```python
from build123d import *

# Parameters (mm, degrees)
SKETCH1_W                                           = 60
SKETCH1_H                                           = 100
BOSS_EXTRUDE1_DEPTH                                 = 8
CBORE_FOR_M6_HEX_SOCKET_HEAD_CAP_SCREW1_D           = 6.6
CBORE_FOR_M6_HEX_SOCKET_HEAD_CAP_SCREW1_CBORE_D     = 11
CBORE_FOR_M6_HEX_SOCKET_HEAD_CAP_SCREW1_CBORE_DEPTH = 6.4
SKETCH6_R                                           = 14.05
CUT_EXTRUDE1_DEPTH                                  = 61.464865831
SKETCH7_W                                           = 60
SKETCH7_H                                           = 16
BOSS_EXTRUDE2_DEPTH                                 = 32
CBORE_FOR_M6_HEX_SOCKET_HEAD_CAP_SCREW2_D           = 6.6
CBORE_FOR_M6_HEX_SOCKET_HEAD_CAP_SCREW2_CBORE_D     = 11
CBORE_FOR_M6_HEX_SOCKET_HEAD_CAP_SCREW2_CBORE_DEPTH = 6.4


with BuildPart() as part:
    # Sketch1 → Boss-Extrude1 (new, symmetric)
    with BuildSketch(Plane.XY):
        Rectangle(SKETCH1_W, SKETCH1_H)
    extrude(amount=BOSS_EXTRUDE1_DEPTH, both=True)

    # CBORE for M6 Hex Socket Head Cap Screw1 (through all)
    with Locations(Plane.XY.offset(8)):
        with Locations((-20, 40), (20, 40), (20, 0), (-20, 0)):
            CounterBoreHole(CBORE_FOR_M6_HEX_SOCKET_HEAD_CAP_SCREW1_D / 2, CBORE_FOR_M6_HEX_SOCKET_HEAD_CAP_SCREW1_CBORE_D / 2, CBORE_FOR_M6_HEX_SOCKET_HEAD_CAP_SCREW1_CBORE_DEPTH)

    # Sketch6 → Cut-Extrude1 (cut, through all)
    with BuildSketch(Plane.XY.offset(8)):
        with Locations((0, 20)):
            Circle(SKETCH6_R)
    extrude(amount=-CUT_EXTRUDE1_DEPTH, mode=Mode.SUBTRACT)

    # Sketch7 → Boss-Extrude2 (add)
    with BuildSketch(Plane.XY.offset(8)):
        with Locations((0, -42)):
            Rectangle(SKETCH7_W, SKETCH7_H)
    extrude(amount=BOSS_EXTRUDE2_DEPTH)

    # CBORE for M6 Hex Socket Head Cap Screw2 (through all)
    with Locations(Plane(origin=(0, -34, 0), x_dir=(1, 0, 0), z_dir=(0, 1, 0))):
        with Locations((-20, -18), (20, -18), (20, -33), (-20, -33)):
            CounterBoreHole(CBORE_FOR_M6_HEX_SOCKET_HEAD_CAP_SCREW2_D / 2, CBORE_FOR_M6_HEX_SOCKET_HEAD_CAP_SCREW2_CBORE_D / 2, CBORE_FOR_M6_HEX_SOCKET_HEAD_CAP_SCREW2_CBORE_DEPTH)


solid = part.part
```
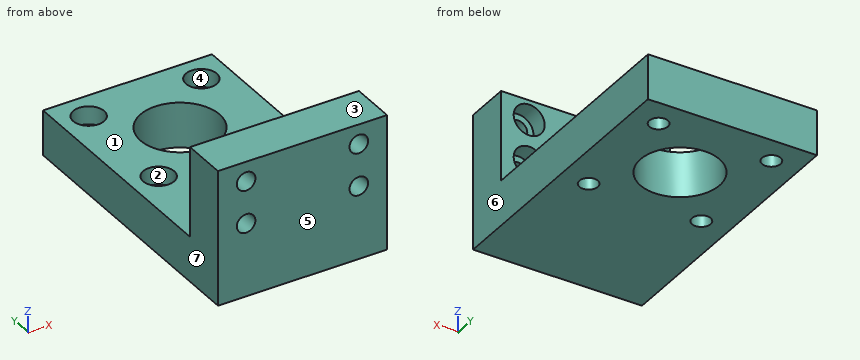
Geometry: final body of the model. Coordinates: model frame, mm. Face numbers are marked on the shaded views. A direction names the side the tool comes from. Round coordinates to 2 decimals unless told otherwise and drop trailing zeros. Write each loop counter-clockwise with the first axis right and the second up, starting at its lowest first coordinate (ties: lowest second). Pieces come first, ordered by that corner, then holes. Notation, with made-up numbers: (-6, 9.5) -> (52, 9.5) arc R13 ccw to (52, 17.5) -> close; hole circle Ø8 at (13, 35). An arc over 180 degrees is marked (long way). Return JSON: item names as keys, results as strings.
Q1. Set-up query: the marked faces 1, 2 and 3. Return all of +Z, -Z, +X, -X, +Y, -Y with unobstructed straight access to the full face (end or side cutting, diameter ignored); none if empty.
From the geometry:
{"face 1": "+Z, +X, -X, +Y", "face 2": "+Z", "face 3": "+Z, +X, -X, +Y, -Y"}
Q2. Ray query, line 1 (X direction, y = -39, z = 18); line 2 (Z direction, x = 20, y = -36.75); line 3 (Z direction, x = 20, y = -43.75). Return the intervals inside material, ascending.
From the geometry:
{"line 1": "-30 to -25.5, -14.5 to 14.5, 25.5 to 30", "line 2": "-8 to 12.5, 23.5 to 27.5, 38.5 to 40", "line 3": "-8 to 14.7, 21.3 to 29.7, 36.3 to 40"}
Q3. Section C-C on z = 18. Return the cut outline in (x, y).
From the geometry:
{"outline": "(-30, -50) -> (-23.3, -50) -> (-23.3, -40.4) -> (-25.5, -40.4) -> (-25.5, -34) -> (-30, -34) -> close; (-16.7, -50) -> (16.7, -50) -> (16.7, -40.4) -> (14.5, -40.4) -> (14.5, -34) -> (-14.5, -34) -> (-14.5, -40.4) -> (-16.7, -40.4) -> close; (23.3, -50) -> (30, -50) -> (30, -34) -> (25.5, -34) -> (25.5, -40.4) -> (23.3, -40.4) -> close"}
Q4. Section A-A on x = 0. Return the cut outline in (y, z), and give its area (3 significant figures).
From the geometry:
{"outline": "(-50, -8) -> (5.95, -8) -> (5.95, 8) -> (-34, 8) -> (-34, 40) -> (-50, 40) -> close; (34.05, -8) -> (50, -8) -> (50, 8) -> (34.05, 8) -> close", "area": "1,660 mm2"}
Q5. Section D-D on y = 24. Return the cut outline in (x, z), and give its area (3 significant figures).
From the geometry:
{"outline": "(-30, -8) -> (-13.47, -8) -> (-13.47, 8) -> (-30, 8) -> close; (13.47, -8) -> (30, -8) -> (30, 8) -> (13.47, 8) -> close", "area": "529 mm2"}
Q6. Mould query, pull axis X, two halves, no side actions, for the marked faces 4, 5, 6 and 7. Classes: +X half, -X half, draft (parallel to the pull), parting line (faces both ways), or undercut.
From the geometry:
{"face 4": "undercut", "face 5": "draft", "face 6": "+X half", "face 7": "-X half"}
Q7. Section B-B on y = 40. Return the cut outline in (x, z).
From the geometry:
{"outline": "(-30, -8) -> (-23.3, -8) -> (-23.3, 1.6) -> (-25.5, 1.6) -> (-25.5, 8) -> (-30, 8) -> close; (-16.7, -8) -> (16.7, -8) -> (16.7, 1.6) -> (14.5, 1.6) -> (14.5, 8) -> (-14.5, 8) -> (-14.5, 1.6) -> (-16.7, 1.6) -> close; (23.3, -8) -> (30, -8) -> (30, 8) -> (25.5, 8) -> (25.5, 1.6) -> (23.3, 1.6) -> close"}
Q8. First-contact query: pin 1 Ø5.5 at (x, z) = (-22, 30.5) entering from +Y; pin 2 Ø4 at (x, z) = (20, 18) entering from -Y; pin 3 Ø6 at (x, y) = (-9, -18.5) entering from +Z; pin 4 Ø5.5 at (x, y) = (-21.5, 0) entering from +Z. Flat tips, straight axial feed; report the tip coordinate or a pass-through.
From the geometry:
{"pin 1": "y = -34", "pin 2": "through", "pin 3": "z = 8", "pin 4": "z = 1.6"}
